Geometry: final body of the model. Coordinates: model frame, mm. A direction names the side the tool comes from. Give positions to 0.01 mm unless a question says otherwise; leave off trailing zeros. Loops run counter-clockwise (first coordinate to the right, second up) from the corner with the lowest first, then second, coordinate; pieces in that order, holes last. Notation, with made-up numbers: (76, 66.25) -> (120, 66.25) arc R12 ccw to (120, 70.25) -> close; hole circle Ø9 at (10.25, 19.5). An arc over 180 degrees is marked (long way). One line per question, with ' | ' between items. Start each with the question number.
Item 1: Section A-A on y = -0.85. Return loops of the section in (x, z) (3 decimals).
Item 2: Material intervals for line 1 along X through (y, z) = (-2.8, 36.5) (3 decimals); line 2 along X through (y, z) = (-0.6, 2.5) (3 decimals); line 3 along Z through (x, y) = (-74, -1.5), sorted ascending. Write a range as [from, to].
Item 3: Section D-D on x = -52.5. Return loops of the section in (y, z) (3 decimals), then the cut area to 3 significant figures.
Item 4: Set-up query: faces 1 (the flat face through (-50.8, -2, 35)), 2 (the flat face through (-3.175, -2, 32)), 3 (the flat face through (-123.825, -2, 32)). Return all of +Z, -Z, +X, -X, +Y, -Y with unobstructed straight access to the full face (end or side cutting, diameter ignored); none if empty.
Item 5: Section C-C on z = 4. Return loops of the section in (x, y) (3 decimals).
Item 6: Section B-B on z = 36. Return loops of the section in (x, y) (3 decimals).
Item 7: Pin query (flat end, axial travel): P1, Ø5, axis at x = -76, z = 24, coming from the +Y side; P2, Ø1, axis at x = -125.5, y = -2, coming from the -Z side; P3, Ø1, axis at y = -1.5, z = 9, coming from the -X side (3 decimals); P4, Ø1.6, axis at x = -58, y = -1.5, coming from the +Z side. Return the tip coordinate at first contact, or that it passes through.
from build123d import *

# Parameters (mm, degrees)
F1_DEPTH = 3.175


with BuildPart() as f1:
    # F0 (on Front) → F1 (new body)
    with BuildSketch(Plane.XZ):
        Polygon((-123.825, 0), (-63.5, 0), (-63.5, 31.75), (-76.2, 31.75), (-76.2, 38.1), (-123.825, 38.1), (-123.825, 25.4), (-127, 25.4), (-127, 12.7), (-123.825, 12.7), align=None)
        Polygon((-63.5, 0), (-3.175, 0), (-3.175, 12.7), (0, 12.7), (0, 25.4), (-3.175, 25.4), (-3.175, 38.1), (-50.8, 38.1), (-50.8, 31.75), (-63.5, 31.75), align=None)
    extrude(amount=F1_DEPTH)


solid = f1.part
Result sheet:
1) outline: (-127, 12.7) -> (-123.825, 12.7) -> (-123.825, 0) -> (-3.175, 0) -> (-3.175, 12.7) -> (0, 12.7) -> (0, 25.4) -> (-3.175, 25.4) -> (-3.175, 38.1) -> (-50.8, 38.1) -> (-50.8, 31.75) -> (-76.2, 31.75) -> (-76.2, 38.1) -> (-123.825, 38.1) -> (-123.825, 25.4) -> (-127, 25.4) -> close
2) line 1: x = [-123.825, -76.2], [-50.8, -3.175] | line 2: x = [-123.825, -3.175] | line 3: z = [0, 31.75]
3) outline: (-3.175, 0) -> (0, 0) -> (0, 31.75) -> (-3.175, 31.75) -> close | area: 101 mm²
4) face 1: +Z, +Y, -Y | face 2: +Z, +X, +Y, -Y | face 3: +Z, -X, +Y, -Y
5) outline: (-123.825, -3.175) -> (-3.175, -3.175) -> (-3.175, 0) -> (-123.825, 0) -> close
6) outline: (-123.825, -3.175) -> (-76.2, -3.175) -> (-76.2, 0) -> (-123.825, 0) -> close; (-50.8, -3.175) -> (-3.175, -3.175) -> (-3.175, 0) -> (-50.8, 0) -> close
7) P1: stops at y = 0 | P2: stops at z = 12.7 | P3: stops at x = -123.825 | P4: stops at z = 31.75
